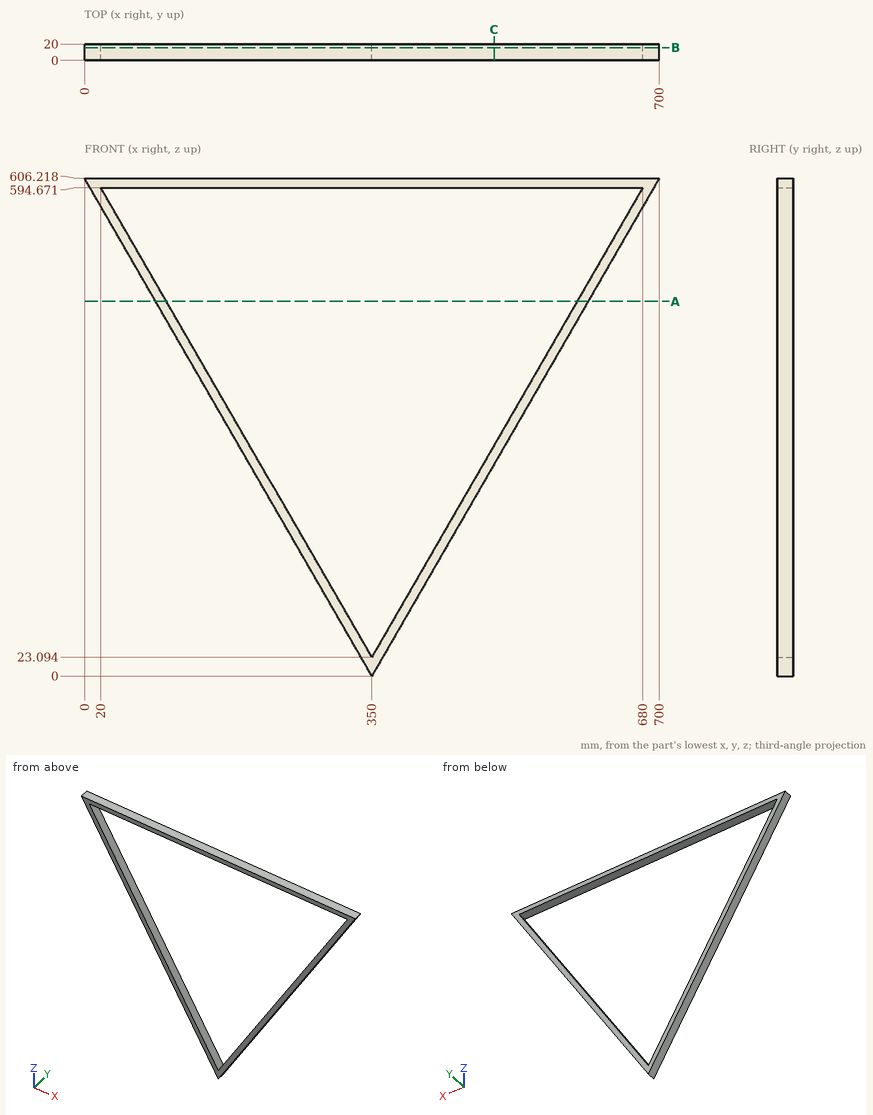
Design review of the part shown in the three views and the two pictorial views. Dimensions are in mm from the part's minimum x, y and z. Give positions to 0.01 mm unless a question says otherwise; leave off trailing zeros. Loops run counter-clockwise (first coordinate to the right, second up) from the corner with the lowest first, then second, coordinate; pieces in that order, holes last. Notation, with made-up numbers: (32, 7) -> (82, 7) arc R22 ccw to (82, 38) -> close; hole circle Ø11 at (-29, -28.5). An arc over 180 degrees is marked (long way). Write each question's results on one line, items separated by ' | '.
1) Insertion check: pin 1 Ø5 at (y, z) = (6, 440.5) entering from -X; pin 2 Ø1 at (y, z) = (8.5, 138.5) entering from -X; pin 3 Ø3 at (y, z) = (11.5, 450.5) entering from +X. Each pin has a flat end and moves straight along its axis. Give the tip position at first contact, or say it passes through.
Conclusion:
pin 1: stops at x = 94.23 | pin 2: stops at x = 269.75 | pin 3: stops at x = 610.96
2) Take a section at C-C, the plane x = 499. Give the boundary of the cut face in (y, z).
Conclusion:
outline: (0, 258.08) -> (20, 258.08) -> (20, 281.17) -> (0, 281.17) -> close; (0, 594.67) -> (20, 594.67) -> (20, 606.22) -> (0, 606.22) -> close
3) Take a section at B-B, the plane y = 15.5. Give the boundary of the cut face in (x, z).
Conclusion:
outline: (0, 606.22) -> (350, 0) -> (700, 606.22) -> close; hole (20, 594.67) -> (350, 23.09) -> (680, 594.67) -> close
4) Take a section at A-A, the plane z = 456.5. Give the boundary of the cut face in (x, y).
Conclusion:
outline: (86.44, 0) -> (99.77, 0) -> (99.77, 20) -> (86.44, 20) -> close; (600.23, 0) -> (613.56, 0) -> (613.56, 20) -> (600.23, 20) -> close
5) For line 1 along X through (y, z) = (18, 398) (1 decimal); line 2 along Z through (x, y) = (473, 17) (1 decimal); line 3 along Z through (x, y) = (587, 15.25) (1 decimal), list the stretches that pass through material, from the lowest coordinate up. Write a range as from..to.
Conclusion:
line 1: x = 120.2..133.5, 566.5..579.8 | line 2: z = 213..236.1, 594.7..606.2 | line 3: z = 410.5..433.6, 594.7..606.2
